Read the model definition and answer for the solid it produces. Units are mm, in the model's axes. A direction names the side the tool comes from. Give positions to 0.01 mm unless a question says otherwise; leave off trailing zeros. Order: outer loops, then holes, each group sorted by start corner. A loop starts at its lowest first (then second) coordinate and runs counter-clockwise, first axis right, second up. Notation, with made-up numbers: (9, 3) -> (46, 3) arc R15 ccw to (46, 22) -> close; hole circle Ø5 at (28, -40). An arc over 180 degrees is marked (long way). Use one line per item in the form item = value.
```python
from build123d import *

# Parameters (mm, degrees)
F1_DEPTH = 20
F2_R     = 2.85
F3_DEPTH = 6.2
F4_W     = 4.34
F4_H     = 4.34
F5_DEPTH = 8.7


with BuildPart() as f1:
    # F0 (on Right) → F1 (new body)
    with BuildSketch(Plane.YZ):
        Polygon((-3, 0), (-3, -6.2), (3, -6.2), (3, 0), (1.85, 0), (-1.85, 0), align=None)
    extrude(amount=-F1_DEPTH)

    # F2 (on face) → F3 (join)
    with BuildSketch(Plane.YZ):
        with Locations((0, -3.1)):
            Circle(F2_R)
    extrude(amount=F3_DEPTH)

    # F4 (on face) → F5 (join)
    with BuildSketch(Plane(origin=(-20, 0, 0), x_dir=(0, -1, 0), z_dir=(-1, 0, 0))):
        with Locations((0, -3.1)):
            Rectangle(F4_W, F4_H)
    extrude(amount=F5_DEPTH)


solid = f1.part
```
Item 1: The part is cut by section B-B on y = 0. Give the vertices of the cut face in (x, z), and give its area (3 significant figures).
Checks:
outline = (-28.7, -5.27) -> (-20, -5.27) -> (-20, -6.2) -> (0, -6.2) -> (0, -5.95) -> (6.2, -5.95) -> (6.2, -0.25) -> (0, -0.25) -> (0, 0) -> (-20, 0) -> (-20, -0.93) -> (-28.7, -0.93) -> close
area = 197 mm²
Item 2: Which of the six approach directions +Z, -Z, +X, -X, +Y, -Y give full straight-line access (tool end or side, diameter ignored) to faces 1 (the cylindrical face through (3.057, -0.371, -0.274)), 2 (the flat face through (-24, 0, -5.27)), 3 (the flat face through (-24, -2.17, -3)), 4 (the flat face through (-24, 0, -0.93)), 5 (the flat face through (-24, 2.17, -3))?
Checks:
face_1 = +X
face_2 = -Z, -X, +Y, -Y
face_3 = +Z, -Z, -X, -Y
face_4 = +Z, -X, +Y, -Y
face_5 = +Z, -Z, -X, +Y
Item 3: The part is cut by section A-A on z = -3.1. Give the vertices of the cut face in (x, y).
Checks:
outline = (-28.7, -2.17) -> (-20, -2.17) -> (-20, -3) -> (0, -3) -> (0, -2.85) -> (6.2, -2.85) -> (6.2, 2.85) -> (0, 2.85) -> (0, 3) -> (-20, 3) -> (-20, 2.17) -> (-28.7, 2.17) -> close
Item 4: Given pin 1 Ø2 at (x, z) = (-22.5, -2) entering from -Y; pin 2 Ø1.3 at (x, y) = (-24.5, 0.5) entering from -Z, each flat-ended and moving along its own axis, determine where each tip first touches the part or whether it passes through.
Checks:
pin_1 = -2.17
pin_2 = -5.27
Item 5: Straight lines are drawn through the part: L1, parallel to Y at x = 1.5, z = -1.25; L2, parallel to X at y = -2.4, z = -2; L3, parallel to Y at x = 1.5, z = -3. For each, find the intervals that lie inside material, in ascending order. Write a range as from..to.
Checks:
L1 = -2.17..2.17
L2 = -20..6.2
L3 = -2.85..2.85
Item 6: The part is cut by section C-C on x = -25.5. Give the vertices of the cut face in (y, z).
Checks:
outline = (-2.17, -5.27) -> (2.17, -5.27) -> (2.17, -0.93) -> (-2.17, -0.93) -> close
